Could you check a few things on this model? Use its own coordinates, in mm. A direction names the side the tool comes from. Give positions to 0.01 mm unless a question says otherwise; leave off trailing zeros. Loops run counter-clockwise (first coordinate to the right, second up) from the corner with the lowest first, then second, coordinate; pieces in that order, holes last. Notation, with made-up numbers: (-38.5, 27) - (-18.5, 27) arc R16 ccw to (-18.5, 47) - close; hole circle Ø9 at (5.25, 54). An arc over 180 degrees is marked (long way). Use CSV: the item, a comma, the result in double quotes.
from build123d import *

# Parameters (mm, degrees)
BOSS_EXTRUDE1_DEPTH = 24
SKETCH2_R           = 5
CUT_EXTRUDE1_DEPTH  = 100.477304276
CUT_EXTRUDE2_DEPTH  = 100.477304276
FILLET1_R           = 6


with BuildPart() as part:
    # Sketch1 → Boss-Extrude1 (new body)
    with BuildSketch(Plane.XY):
        with BuildLine():
            Line((0, 10), (0, 54.457793632))
            ThreePointArc((0, 54.457793632), (5.821431905, 63.542922617), (16.507913735, 62.050359656))
            Line((16.507913735, 62.050359656), (68.375339639, 17.592566024))
            ThreePointArc((68.375339639, 17.592566024), (71.246276054, 6.530537523), (61.867425905, 0))
            Line((61.867425905, 0), (10, 0))
            ThreePointArc((10, 0), (2.928932188, 2.928932188), (0, 10))
        make_face()
    extrude(amount=BOSS_EXTRUDE1_DEPTH)

    # Sketch2 → Cut-Extrude1 (cut, through all)
    with BuildSketch(Plane.XY.offset(24)):
        with Locations((10, 54.457793632)):
            Circle(SKETCH2_R)
        with Locations((61.867425905, 10)):
            Circle(SKETCH2_R)
    extrude(amount=-CUT_EXTRUDE1_DEPTH, mode=Mode.SUBTRACT)

    # Sketch3 → Cut-Extrude2 (cut, through all)
    with BuildSketch(Plane(origin=(0, 0, 0), x_dir=(-1, 0, 0), z_dir=(0, 0, -1))):
        with BuildLine():
            Line((0, 0), (-20, 0))
            Line((-20, 0), (-20, 14))
            ThreePointArc((-20, 14), (-18.242640687, 18.242640687), (-14, 20))
            Line((-14, 20), (0, 20))
            Line((0, 20), (0, 0))
        make_face()
    extrude(amount=-CUT_EXTRUDE2_DEPTH, mode=Mode.SUBTRACT)

    # Fillet1
    fillet1_edges = [part.edges().sort_by_distance(p)[0] for p in [
        (0, 20, 12),
        (20, 0, 12),
    ]]
    fillet(fillet1_edges, radius=FILLET1_R)


solid = part.part
1) I need wall thicknesses on line 1 along Y through (x, z) = (10, 13.5); line 2 along X through (y, z) = (51, 4.75); line 3 along Y through (x, z) = (59, 12.5). Which ranges of each line are inside material? Lowest first, please.
Answer below:
line 1,"y = 20 to 49.46, 59.46 to 64.46"
line 2,"x = 0 to 6.39, 13.61 to 29.4"
line 3,"y = 0 to 5.9, 14.1 to 25.63"
2) I'm going to push flat-ended pins straight in: P1, Ø2.5, axis at x = 10.5, z = 12, coming from the -Y side; P2, Ø8, axis at x = 20, z = 13.5, coming from the +Y side; P3, Ø1.5, axis at y = 51.5, z = 12, coming from the +X side; P4, Ø13, axis at x = 61.87, y = 10, coming from the -Z side. Where does each tip first touch, or does it pass through?
Answer below:
P1,"stops at y = 20"
P2,"stops at y = 62.46"
P3,"stops at x = 29.69"
P4,"stops at z = 0"
3) Suppose I cut it at A-A (y = 10). Please give me the cut outline in (x, z), plus the area to 3 significant figures.
Answer below:
outline,"(20, 0) - (56.87, 0) - (56.87, 24) - (20, 24) - close; (66.87, 0) - (71.87, 0) - (71.87, 24) - (66.87, 24) - close"
area,"1,000 mm2"
4) Suppose I cut it at C-C (z = 16.75). Please give me the cut outline in (x, y).
Answer below:
outline,"(0, 26) arc R6 ccw to (6, 20) - (14, 20) arc R6 cw to (20, 14) - (20, 6) arc R6 ccw to (26, 0) - (61.87, 0) arc R10 ccw to (68.38, 17.59) - (16.51, 62.05) arc R10 ccw to (0, 54.46) - close; hole circle Ø10 at (10, 54.46); hole circle Ø10 at (61.87, 10)"
5) Suppose I cut it at D-D (y = 45). Please give me the cut outline in (x, z), plus the area to 3 significant figures.
Answer below:
outline,"(0, 0) - (36.4, 0) - (36.4, 24) - (0, 24) - close"
area,"874 mm2"
6) Suppose I cut it at B-B (x = 10). Please give me the cut outline in (y, z), plus the area to 3 significant figures.
Answer below:
outline,"(20, 0) - (49.46, 0) - (49.46, 24) - (20, 24) - close; (59.46, 0) - (64.46, 0) - (64.46, 24) - (59.46, 24) - close"
area,"827 mm2"
7) We'd pull the mould along X, two halves only. Please class faces 1 (the cylindrical face through (9.349, 59.415, 12.168)), 2 (the cylindrical face through (66.637, 11.502, 12.168)), 3 (the flat face through (28, 26, 24)), 4 (the flat face through (20, 10, 12)): +X half, -X half, draft (parallel to the pull), parting line (faces both ways), or undercut.
Answer below:
face 1,"undercut"
face 2,"undercut"
face 3,"draft"
face 4,"-X half"
8) Which directions (+Z, -Z, +X, -X, +Y, -Y) give clear straight access to the entire face, cutting with the end or side of a thin tool? Please do faces 5 (the flat face through (10, 20, 12)), 6 (the flat face through (44, 0, 12)).
Answer below:
face 5,"+Z, -Z, -X, -Y"
face 6,"+Z, -Z, +X, -X, -Y"
